Here's how the part is built. I have some questions about the finished solid (model axes, mm). A direction names the side the tool comes from. Round coordinates to 2 decimals unless told otherwise and drop trailing zeros. Write each loop counter-clockwise with the first axis right and the second up, starting at its lowest first coordinate (ties: lowest second). Pieces come first, ordered by that corner, then holes. Notation, with made-up numbers: (49.5, -34) - (106.5, -34) arc R12 ccw to (106.5, -29) - close; hole circle Ø6 at (1, 58.25). An arc over 180 degrees is marked (long way). Return JSON: item names as keys, results as strings. Group by question number.
Autodesk Fusion 360 part; units mm, degrees
sketch "スケッチ1" plane through (0, 0, 0) normal (0, 0, 1) x (1, 0, 0)
  circle A0 centre (0, 0) radius 3
  line L0 (0, 0) -> (-4, 0)
  circle A1 centre (-4, 0) radius 9
  circle A2 centre (0, 0) radius 4
  dimension "d1" = 6
  dimension "d2" = 4
  dimension "d3" = 18
  dimension "d14" = 8
extrude "押し出し1" add sketch "スケッチ1" against normal blind 10 contours A0
extrude "押し出し2" add sketch "スケッチ1" along normal blind 17 contours A0 | A2 | A1
sketch "スケッチ2" plane through (0, 0, 17) normal (0, 0, 1) x (1, 0, 0)
  circle A0 centre (-4, 0) radius 9
  circle A1 centre (0, 0) radius 3
  circle A2 centre (0, 0) radius 4
  dimension "d8" = 6
  dimension "d11" = 8
extrude "押し出し3" add sketch "スケッチ2" along normal blind 10 contours A1
extrude "押し出し4" add sketch "スケッチ2" along normal blind 1.5 contours A2
extrude "押し出し5" add sketch "スケッチ1" against normal blind 1.5 contours A2
extrude "押し出し6" cut sketch "スケッチ2" against normal blind 5 contours A0
extrude "押し出し7" cut 1 faces at (3.6406, -0.3478, 18.5) along direction (0, 0, -1) blind 5
extrude "押し出し8" cut 1 faces at (-9.9665, 0.4471, 12) along direction (0, 0, -1) blind 3.5
extrude "押し出し9" cut 1 faces at (3.6406, -0.3478, 13.5) along direction (0, 0, -1) blind 3.5
extrude "押し出し10" cut 1 faces at (0.3505, -0.866, 27) along direction (0, 0, -1) blind 5
extrude "押し出し11" add 1 faces at (3.6406, -0.3478, 10) along direction (0, 0, 1) blind 5
extrude "押し出し12" cut 1 faces at (-9.9665, 0.4471, 8.5) along direction (0, 0, -1) blind 1.5
extrude "押し出し13" add 1 faces at (-9.9665, 0.4471, 7) along direction (0, 0, 1) blind 1
extrude "押し出し14" cut 1 faces at (3.6406, -0.3478, 15) along direction (0, 0, -1) blind 6.5
extrude "押し出し15" add 1 faces at (3.6406, -0.3478, 8.5) along direction (0, 0, 1) blind 0.5
extrude "押し出し16" cut 1 faces at (3.6406, -0.3478, 9) along direction (0, 0, -1) blind 0.5
extrude "押し出し17" add 1 faces at (3.6406, -0.3478, 8.5) along direction (0, 0, 1) blind 0.5
sketch "スケッチ3" plane through (0, 0, 0) normal (0, 0, 1) x (1, 0, 0)
  circle A0 centre (-4, 0) radius 11
  circle A1 centre (-4, 0) radius 9
  dimension "d41" = 22
extrude "押し出し18" add sketch "スケッチ3" against normal blind 1 contours A0 | A1
extrude "押し出し19" add 1 faces at (3.6406, -0.3478, 9) along direction (0, 0, 1) blind 2
extrude "押し出し20" add 1 faces at (-9.9665, 0.4471, 8) along direction (0, 0, 1) blind 2
extrude "押し出し21" cut 1 faces at (3.6406, -0.3478, 11) along direction (0, 0, -1) blind 1
extrude "押し出し22" cut 1 faces at (-9.6332, 0.4471, 10) along direction (0, 0, -1) blind 1
sketch "スケッチ4" plane through (0, 0, 9) normal (0, 0, 1) x (1, 0, 0)
  circle A0 centre (0, 0) radius 3
  circle A1 centre (-4, 0) radius 9
  circle A2 centre (0, 0) radius 3.75
  dimension "d52" = 7.5
extrude "押し出し23" add sketch "スケッチ4" along normal blind 0.5 contours A2
1) I need wall thicknesses on line 1 along Z through (x, y) = (-6.25, 0.75); line 2 along Z through (x, y) = (-7, 9); line 3 along X through (y, z) = (2.75, -3.5). Which ranges of each line are inside material? Lowest first, please.
2) Imagine slicing it at C-C (z = 14). Please give me the cut outline in (x, y), plus the area to 3 significant figures.
3) Imagine slicing it at B-B (x = -8.75). Please give me the cut outline in (y, z), plus the area to 3 significant figures.
4) For faces 1 (the cylindrical face through (6.161, -4.213, -0.493)), 2 (the cylindrical face through (-0.867, -3.905, -1.246)), 3 (the cylindrical face through (-3, 0, 16)), which set-ups out of +Z, -Z, +X, -X, +Y, -Y let a thin tool reach every point of the face, with its end or its side?
5) Imagine slicing it at A-A (y = 0). Please give me the cut outline in (x, z).
6) Imagine slicing it at D-D (x = 0). Please give me the cut outline in (y, z).
7) Will these pins go through, and if not, where does the flat tip stop? pin 1 Ø2 at (x, y) = (-8.5, 6.5) entering from +Z; pin 2 Ø4 at (y, z) = (2, 14) entering from +X; pin 3 Ø1 at (x, y) = (4.5, 7) entering from -Z.
Results found:
{
 "1": {"line 1": "z = -1 to 9", "line 2": "z = -1 to 0", "line 3": "x = -1.2 to 1.2"},
 "2": {"outline": "circle Ø6 at (0, 0)", "area": "28.3 mm²"},
 "3": {"outline": "(-9.92, -1) - (9.92, -1) - (9.92, 0) - (7.64, 0) - (7.64, 9) - (-7.64, 9) - (-7.64, 0) - (-9.92, 0) - close", "area": "157 mm²"},
 "4": {"face 1": "+Z, -Z", "face 2": "-Z", "face 3": "+Z"},
 "5": {"outline": "(-15, -1) - (-4, -1) - (-4, -1.5) - (-3, -1.5) - (-3, -10) - (3, -10) - (3, -1.5) - (4, -1.5) - (4, -1) - (7, -1) - (7, 0) - (5, 0) - (5, 9) - (3.75, 9) - (3.75, 9.5) - (3, 9.5) - (3, 22) - (-3, 22) - (-3, 9.5) - (-3.75, 9.5) - (-3.75, 9) - (-13, 9) - (-13, 0) - (-15, 0) - close"},
 "6": {"outline": "(-10.25, -1) - (-4, -1) - (-4, -1.5) - (-3, -1.5) - (-3, -10) - (3, -10) - (3, -1.5) - (4, -1.5) - (4, -1) - (10.25, -1) - (10.25, 0) - (8.06, 0) - (8.06, 9) - (3.75, 9) - (3.75, 9.5) - (3, 9.5) - (3, 22) - (-3, 22) - (-3, 9.5) - (-3.75, 9.5) - (-3.75, 9) - (-8.06, 9) - (-8.06, 0) - (-10.25, 0) - close"},
 "7": {"pin 1": "stops at z = 9", "pin 2": "stops at x = 3", "pin 3": "stops at z = -1"}
}
